Source: CAD feature listing. Evaluate the final solid. Frame: model axes, mm. Give positions to 0.01 mm unless a question says otherwise; leave off trailing zeros. Loops run counter-clockwise (first coordinate to the right, second up) from the corner with the lowest first, then second, coordinate; pieces in that order, holes last. Notation, with made-up numbers: M 8.5,48.5 L 39.5,48.5 A32 cw 39.5,83.5 Z; hole C 57,57 d3. An arc over 180 degrees is marked long. Answer in a Markdown table with one row per item.
```python
from build123d import *

# Parameters (mm, degrees)
SKETCH1_W           = 5
SKETCH1_H           = 8
BOSS_EXTRUDE1_DEPTH = 185
BOSS_EXTRUDE2_DEPTH = 200
SKETCH3_W           = 5
SKETCH3_H           = 8
CUT_EXTRUDE1_DEPTH  = 200
CUT_EXTRUDE2_REACH  = 202.176
SKETCH4_R           = 1
SKETCH5_R           = 1.9
CUT_EXTRUDE3_DEPTH  = 2
CHAMFER1_SIZE       = 0.5
CHAMFER2_SIZE       = 0.5
CUT_EXTRUDE4_DEPTH  = 5


with BuildPart() as part:
    # Sketch1 → Boss-Extrude1 (new body)
    with BuildSketch(Plane.XY):
        Rectangle(SKETCH1_W, SKETCH1_H)
    extrude(amount=BOSS_EXTRUDE1_DEPTH)

    # Sketch2 → Boss-Extrude2 (add)
    with BuildSketch(Plane(origin=(0, 0, 0), x_dir=(-1, 0, 0), z_dir=(0, 0, -1))):
        with BuildLine():
            Line((-2.5, 4), (-2.5, 1.798202453))
            ThreePointArc((-2.5, 1.798202453), (-2.423157727, 1.350663613), (-2.2014329, 0.954388646))
            ThreePointArc((-2.2014329, 0.954388646), (-1.511468603, -0.151015487), (-2.5, -1))
            Line((-2.5, -1), (-2.5, -4))
            Line((-2.5, -4), (2.5, -4))
            Line((2.5, -4), (2.5, -1))
            ThreePointArc((2.5, -1), (1.511468603, -0.151015487), (2.2014329, 0.954388646))
            ThreePointArc((2.2014329, 0.954388646), (2.423157727, 1.350663613), (2.5, 1.798202453))
            Line((2.5, 1.798202453), (2.5, 4))
            Line((2.5, 4), (-2.5, 4))
        make_face()
    extrude(amount=BOSS_EXTRUDE2_DEPTH)

    # Sketch3 → Cut-Extrude1 (cut)
    with BuildSketch(Plane.XY.offset(185)):
        Rectangle(SKETCH3_W, SKETCH3_H)
    extrude(amount=-CUT_EXTRUDE1_DEPTH, mode=Mode.SUBTRACT)

    # Sketch4 → Cut-Extrude2 (cut, up to next)
    with BuildSketch(Plane.XZ.offset(4), mode=Mode.PRIVATE) as cut_extrude2_sk1:
        with Locations(Location((0, -35, 0), (0, 0, 270))):
            Circle(SKETCH4_R)
    cut_extrude2_tool1 = extrude(cut_extrude2_sk1.sketch, amount=-CUT_EXTRUDE2_REACH, mode=Mode.PRIVATE) & part.part
    # Sketch4 → Cut-Extrude2 (cut, up to next)
    with BuildSketch(Plane.XZ.offset(4), mode=Mode.PRIVATE) as cut_extrude2_sk2:
        with Locations(Location((0, -55, 0), (0, 0, 270))):
            Circle(SKETCH4_R)
    cut_extrude2_tool2 = extrude(cut_extrude2_sk2.sketch, amount=-CUT_EXTRUDE2_REACH, mode=Mode.PRIVATE) & part.part
    # Sketch4 → Cut-Extrude2 (cut, up to next)
    with BuildSketch(Plane.XZ.offset(4), mode=Mode.PRIVATE) as cut_extrude2_sk3:
        with Locations(Location((0, -75, 0), (0, 0, 270))):
            Circle(SKETCH4_R)
    cut_extrude2_tool3 = extrude(cut_extrude2_sk3.sketch, amount=-CUT_EXTRUDE2_REACH, mode=Mode.PRIVATE) & part.part
    # Sketch4 → Cut-Extrude2 (cut, up to next)
    with BuildSketch(Plane.XZ.offset(4), mode=Mode.PRIVATE) as cut_extrude2_sk4:
        with Locations(Location((0, -95, 0), (0, 0, 270))):
            Circle(SKETCH4_R)
    cut_extrude2_tool4 = extrude(cut_extrude2_sk4.sketch, amount=-CUT_EXTRUDE2_REACH, mode=Mode.PRIVATE) & part.part
    # Sketch4 → Cut-Extrude2 (cut, up to next)
    with BuildSketch(Plane.XZ.offset(4), mode=Mode.PRIVATE) as cut_extrude2_sk5:
        with Locations(Location((0, -115, 0), (0, 0, 270))):
            Circle(SKETCH4_R)
    cut_extrude2_tool5 = extrude(cut_extrude2_sk5.sketch, amount=-CUT_EXTRUDE2_REACH, mode=Mode.PRIVATE) & part.part
    # Sketch4 → Cut-Extrude2 (cut, up to next)
    with BuildSketch(Plane.XZ.offset(4), mode=Mode.PRIVATE) as cut_extrude2_sk6:
        with Locations(Location((0, -135, 0), (0, 0, 270))):
            Circle(SKETCH4_R)
    cut_extrude2_tool6 = extrude(cut_extrude2_sk6.sketch, amount=-CUT_EXTRUDE2_REACH, mode=Mode.PRIVATE) & part.part
    # Sketch4 → Cut-Extrude2 (cut, up to next)
    with BuildSketch(Plane.XZ.offset(4), mode=Mode.PRIVATE) as cut_extrude2_sk7:
        with Locations(Location((0, -155, 0), (0, 0, 270))):
            Circle(SKETCH4_R)
    cut_extrude2_tool7 = extrude(cut_extrude2_sk7.sketch, amount=-CUT_EXTRUDE2_REACH, mode=Mode.PRIVATE) & part.part
    # Sketch4 → Cut-Extrude2 (cut, up to next)
    with BuildSketch(Plane.XZ.offset(4), mode=Mode.PRIVATE) as cut_extrude2_sk8:
        with Locations(Location((0, -175, 0), (0, 0, 270))):
            Circle(SKETCH4_R)
    cut_extrude2_tool8 = extrude(cut_extrude2_sk8.sketch, amount=-CUT_EXTRUDE2_REACH, mode=Mode.PRIVATE) & part.part
    # Sketch4 → Cut-Extrude2 (cut, up to next)
    with BuildSketch(Plane.XZ.offset(4), mode=Mode.PRIVATE) as cut_extrude2_sk9:
        with Locations(Location((0, -195, 0), (0, 0, 270))):
            Circle(SKETCH4_R)
    cut_extrude2_tool9 = extrude(cut_extrude2_sk9.sketch, amount=-CUT_EXTRUDE2_REACH, mode=Mode.PRIVATE) & part.part
    add(cut_extrude2_tool1.solids().sort_by_distance((0, -4, -35))[0], mode=Mode.SUBTRACT)
    add(cut_extrude2_tool2.solids().sort_by_distance((0, -4, -55))[0], mode=Mode.SUBTRACT)
    add(cut_extrude2_tool3.solids().sort_by_distance((0, -4, -75))[0], mode=Mode.SUBTRACT)
    add(cut_extrude2_tool4.solids().sort_by_distance((0, -4, -95))[0], mode=Mode.SUBTRACT)
    add(cut_extrude2_tool5.solids().sort_by_distance((0, -4, -115))[0], mode=Mode.SUBTRACT)
    add(cut_extrude2_tool6.solids().sort_by_distance((0, -4, -135))[0], mode=Mode.SUBTRACT)
    add(cut_extrude2_tool7.solids().sort_by_distance((0, -4, -155))[0], mode=Mode.SUBTRACT)
    add(cut_extrude2_tool8.solids().sort_by_distance((0, -4, -175))[0], mode=Mode.SUBTRACT)
    add(cut_extrude2_tool9.solids().sort_by_distance((0, -4, -195))[0], mode=Mode.SUBTRACT)

    # Sketch5 → Cut-Extrude3 (cut)
    with BuildSketch(Plane(origin=(0, 4, 0), x_dir=(1, 0, 0), z_dir=(0, 1, 0))):
        with Locations(Location((0, 195, 0), (0, 0, 180))):
            Circle(SKETCH5_R)
        with Locations(Location((0, 175, 0), (0, 0, 180))):
            Circle(SKETCH5_R)
        with Locations(Location((0, 155, 0), (0, 0, 180))):
            Circle(SKETCH5_R)
        with Locations(Location((0, 135, 0), (0, 0, 180))):
            Circle(SKETCH5_R)
        with Locations(Location((0, 115, 0), (0, 0, 180))):
            Circle(SKETCH5_R)
        with Locations(Location((0, 95, 0), (0, 0, 180))):
            Circle(SKETCH5_R)
        with Locations(Location((0, 75, 0), (0, 0, 180))):
            Circle(SKETCH5_R)
        with Locations(Location((0, 55, 0), (0, 0, 180))):
            Circle(SKETCH5_R)
        with Locations(Location((0, 35, 0), (0, 0, 180))):
            Circle(SKETCH5_R)
    extrude(amount=-CUT_EXTRUDE3_DEPTH, mode=Mode.SUBTRACT)

    # Chamfer1
    chamfer1_edges = [part.edges().sort_by_distance(p)[0] for p in [
        (-2.5, 4, -107.5),
    ]]
    chamfer(chamfer1_edges, length=CHAMFER1_SIZE)

    # Chamfer2
    chamfer2_edges = [part.edges().sort_by_distance(p)[0] for p in [
        (2.5, 4, -107.5),
    ]]
    chamfer(chamfer2_edges, length=CHAMFER2_SIZE)

    # Sketch6 → Cut-Extrude4 (cut)
    with BuildSketch(Plane.XY.offset(-15)):
        with BuildLine():
            Line((2.5, 1.798202453), (2.5, 3.5))
            Line((2.5, 3.5), (2, 4))
            Line((2, 4), (-2, 4))
            Line((-2, 4), (-2.5, 3.5))
            Line((-2.5, 3.5), (-2.5, 1.798202453))
            ThreePointArc((-2.5, 1.798202453), (-2.423157727, 1.350663613), (-2.2014329, 0.954388646))
            ThreePointArc((-2.2014329, 0.954388646), (-1.511468603, -0.151015487), (-2.5, -1))
            Line((-2.5, -1), (-2.5, -4))
            Line((-2.5, -4), (2.5, -4))
            Line((2.5, -4), (2.5, -1))
            ThreePointArc((2.5, -1), (1.511468603, -0.151015487), (2.2014329, 0.954388646))
            ThreePointArc((2.2014329, 0.954388646), (2.423157727, 1.350663613), (2.5, 1.798202453))
        make_face()
    extrude(amount=-CUT_EXTRUDE4_DEPTH, mode=Mode.SUBTRACT)


solid = part.part
```
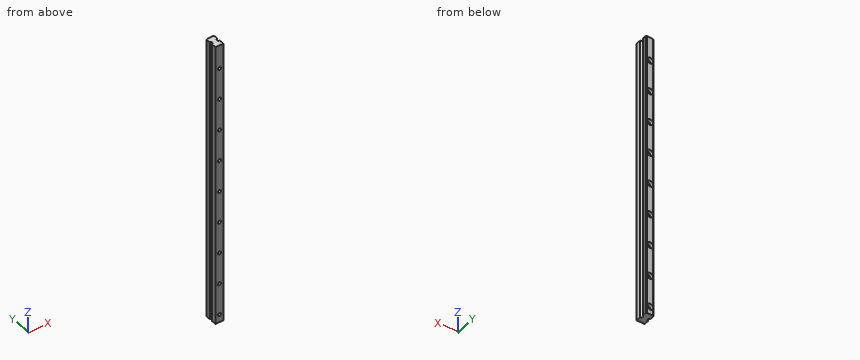
Q1. Contact query for flat-ended pins moving along their axis: pin 1 Ø1.9 at (x, z) = (-0.5, -115.5) entering from +Y; pin 2 Ø1.9 at (x, z) = (0.5, -54) entering from +Y. Output: stop coordinate, or through.
Values follow:
| item | result |
|---|---|
| pin 1 | y = 2 |
| pin 2 | y = 4 |
Q2. Section query A-A (x = 0). Give the number of separate pieces and of enclosed holes in the cut face, plus the area to 3 significant figures.
Values follow:
| item | result |
|---|---|
| separate pieces | 10 |
| enclosed holes | 0 |
| area | 1,260 mm^2 |
Q3. Section query B-B (z = -140.5). Output: boundary loops of the cut face in (x, y), plus the area to 3 significant figures.
Values follow:
| item | result |
|---|---|
| outline | M -2.5,-4 L 2.5,-4 L 2.5,-1 A1 cw 2.2,0.95 A1.34 ccw 2.5,1.8 L 2.5,3.5 L 2,4 L -2,4 L -2.5,3.5 L -2.5,1.8 A1.34 ccw -2.2,0.95 A1 cw -2.5,-1 Z |
| area | 36.5 mm^2 |
Q4. Ray query, probe 1 along X at (y, z) = (-2, -155); probe 2 along X at (y, z) = (2.6, -195); probe 3 along Y at (x, z) = (-1.6, -173). Return the intervals inside material, ascending. Write a range as from..to.
Values follow:
| item | result |
|---|---|
| probe 1 | -2.5..-1, 1..2.5 |
| probe 2 | -2.5..-1.9, 1.9..2.5 |
| probe 3 | -4..-0.44, 0.44..4 |
